Read the model definition and answer for the solid it produces. Units are mm, in the model's axes. Face numbers are marked on the shaded views. Round coordinates to 2 decimals unless told otherwise and drop trailing zeros. Write each loop counter-clockwise with the first axis right and the second up, starting at its lowest first coordinate (ties: lowest second). Pieces come first, ordered by that corner, then holes.
Autodesk Inventor part; units mm, degrees
ref_plane "YZ Plane" through (0, 0, 0) normal (1, 0, 0) x (0, 1, 0)
ref_plane "XZ Plane" through (0, 0, 0) normal (0, 1, 0) x (-1, 0, 0)
ref_plane "XY Plane" through (0, 0, 0) normal (0, 0, 1) x (1, 0, 0)
sketch "Sketch1" plane through (0, 0, 0) normal (0, 0, 1) x (1, 0, 0)
  line L0 (3.175, 0) -> (22.225, 0)
  line L1 (25.4, 3.175) -> (25.4, 22.225)
  line L2 (22.225, 25.4) -> (3.175, 25.4)
  line L3 (0, 22.225) -> (0, 3.175)
  arc A0 (3.175, 25.4) -> (0, 22.225) centre (3.175, 22.225) ccw
  arc A1 (0, 3.175) -> (3.175, 0) centre (3.175, 3.175) ccw
  arc A2 (22.225, 0) -> (25.4, 3.175) centre (22.225, 3.175) ccw
  arc A3 (25.4, 22.225) -> (22.225, 25.4) centre (22.225, 22.225) ccw
  line L4 (3.175, 23.749) -> (22.225, 23.749)
  arc A4 (23.749, 22.225) -> (22.225, 23.749) centre (22.225, 22.225) ccw
  line L5 (23.749, 22.225) -> (23.749, 3.175)
  arc A5 (22.225, 1.651) -> (23.749, 3.175) centre (22.225, 3.175) ccw
  line L6 (22.225, 1.651) -> (3.175, 1.651)
  arc A6 (1.651, 3.175) -> (3.175, 1.651) centre (3.175, 3.175) ccw
  line L7 (1.651, 3.175) -> (1.651, 22.225)
  arc A7 (3.175, 23.749) -> (1.651, 22.225) centre (3.175, 22.225) ccw
  point P0 (0, 0)
  point P1 (25.4, 0)
  point P2 (0, 25.4)
  dimension "d0" = 25.4
  dimension "d1" = 25.4
  dimension "d2" = 3.175
  dimension "d3" = 1.651
extrude "Extrusion1" add sketch "Sketch1" along normal blind 203.2
sketch "Sketch2" plane through (3.175, 25.4, 0) normal (0, 1, 0) x (1, 0, 0)
  line L0 (19.05, -203.2) -> (0, -203.2)
  line L1 (-3.175, 0) -> (22.2557, 0)
  line L2 (-3.175, 0) -> (32.385, 0) construction
  line L3 (22.2557, 0) -> (22.2557, -14.6824)
  line L4 (-3.175, 0) -> (22.2557, -14.6824)
  line L5 (-3.175, 0) -> (-3.175, -203.2) construction
  line L6 (-3.175, -101.6) -> (22.2557, -101.6) construction
  line L7 (-3.175, -203.2) -> (22.2557, -203.2)
  line L8 (22.2557, -203.2) -> (22.2557, -188.5176)
  line L9 (-3.175, -203.2) -> (22.2557, -188.5176)
  point P0 (0, 0)
extrude "Extrusion2" cut sketch "Sketch2" against normal blind 203.2
sketch "Sketch3" plane through (3.175, 25.4, 201.3669) normal (0, 1, 0) x (1, 0, 0)
  line L0 (0, 199.5338) -> (0, 0)
  line L1 (19.05, 188.5353) -> (19.05, 10.9985)
  line L2 (0, 99.7669) -> (19.05, 99.7669) construction
  circle A0 centre (9.525, 99.7669) radius 2.5512
  point P0 (-3.175, 201.3669)
hole "Hole1" at (12.7, 25.4, 101.6) direction (0, -1, 0) diameter 6.35 end through all
properties part number "2f2ao" material "Steel"
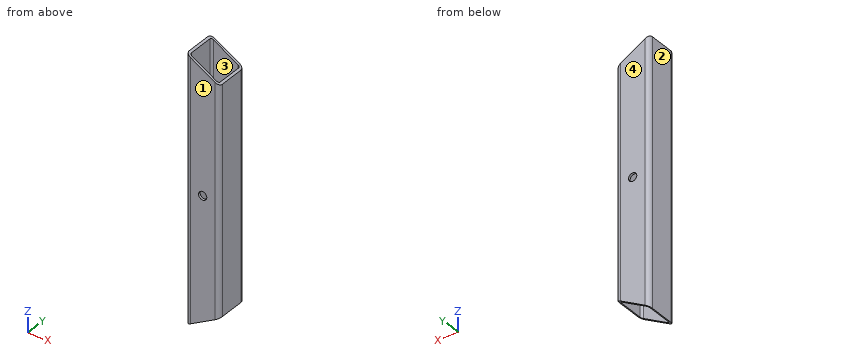
Q1. Determine the mould class of the marked faces 1, 2, 3 and 4 for opening direction Y: pulls with the +Y half, pulls with the -Y half, needs draft (parallel to the pull), parting line crosses it, or undercut.
Verdict:
face 1: pulls with the -Y half
face 2: needs draft
face 3: undercut
face 4: pulls with the +Y half
Q2. Section C-C (z = 48) is taken. Determine the outline of the cut face in (x, y) (3 decimals).
Verdict:
outline: (0, 3.175) arc R3.175 ccw to (3.175, 0) - (22.225, 0) arc R3.175 ccw to (25.4, 3.175) - (25.4, 22.225) arc R3.175 ccw to (22.225, 25.4) - (3.175, 25.4) arc R3.175 ccw to (0, 22.225) - close; hole (1.651, 3.175) arc R1.524 ccw to (3.175, 1.651) - (22.225, 1.651) arc R1.524 ccw to (23.749, 3.175) - (23.749, 22.225) arc R1.524 ccw to (22.225, 23.749) - (3.175, 23.749) arc R1.524 ccw to (1.651, 22.225) - close
Q3. A flat-ended cylindrical pin translates along its axis: pin 1 Ø5 at (x, y) = (21.5, 6.5) entering from -Z. Find the tip coordinate at first contact, or state that the pin passes through.
Verdict:
pin 1: stops at z = 13.71
Q4. Straight lines are drawn through the part: probe 1 along X at (y, z) = (4.5, 64); probe 2 along Z at (x, y) = (12.7, 0.4) (3 decimals). For each, find the intervals that lie inside material, in ascending order.
Verdict:
probe 1: x = 0 to 1.65, 23.75 to 25.4
probe 2: z = 7.332 to 98.425, 104.775 to 195.868
Q5. Section D-D (x = 5.25) is taken. Determine the outline of the cut face in (y, z).
Verdict:
outline: (0, 3.03) - (1.65, 3.03) - (1.65, 200.17) - (0, 200.17) - close; (23.75, 3.03) - (25.4, 3.03) - (25.4, 200.17) - (23.75, 200.17) - close
Q6. Section B-B (z = 101.6) is taken. Determine the outline of the cut face in (x, y) (3 decimals).
Verdict:
outline: (0, 3.175) arc R3.175 ccw to (3.175, 0) - (9.525, 0) - (9.525, 1.651) - (3.175, 1.651) arc R1.524 cw to (1.651, 3.175) - (1.651, 22.225) arc R1.524 cw to (3.175, 23.749) - (9.525, 23.749) - (9.525, 25.4) - (3.175, 25.4) arc R3.175 ccw to (0, 22.225) - close; (15.875, 0) - (22.225, 0) arc R3.175 ccw to (25.4, 3.175) - (25.4, 22.225) arc R3.175 ccw to (22.225, 25.4) - (15.875, 25.4) - (15.875, 23.749) - (22.225, 23.749) arc R1.524 cw to (23.749, 22.225) - (23.749, 3.175) arc R1.524 cw to (22.225, 1.651) - (15.875, 1.651) - close
Q7. Section A-A (y = 16.5) is taken. Determine the outline of the cut face in (x, z).
Verdict:
outline: (0, 0) - (1.65, 0.95) - (1.65, 202.25) - (0, 203.2) - close; (23.75, 13.71) - (25.4, 14.66) - (25.4, 188.54) - (23.75, 189.49) - close
